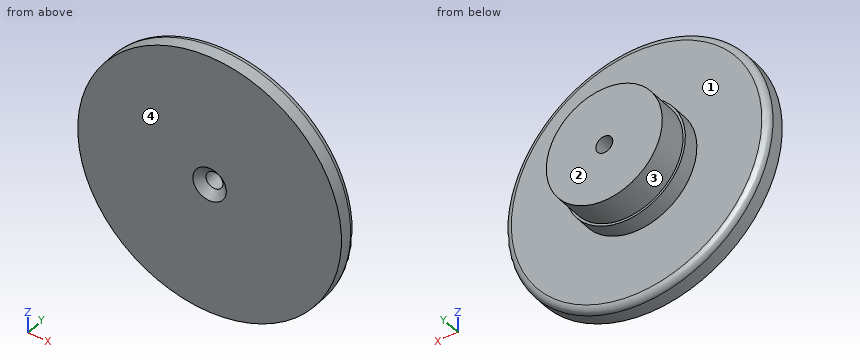
```python
from build123d import *

# Parameters (mm, degrees)
SKETCH1_R                                           = 50.8
SKETCH1_R_2                                         = 23.241
BOSS_EXTRUDE4_DEPTH                                 = 7.62
SKETCH1_6_R                                         = 23.241
SKETCH1_6_R_2                                       = 22.352
BOSS_EXTRUDE5_DEPTH                                 = 13.97
SKETCH1_7_R                                         = 22.352
BOSS_EXTRUDE6_DEPTH                                 = 25.4
CSK_FOR_1_4_FLAT_HEAD_MACHINE_SCREW_100_D           = 6.5278
CSK_FOR_1_4_FLAT_HEAD_MACHINE_SCREW_100_CSINK_D     = 12.8778
CSK_FOR_1_4_FLAT_HEAD_MACHINE_SCREW_100_CSINK_ANGLE = 100
FILLET3_R                                           = 2.54


with BuildPart() as part:
    # Sketch1 → Boss-Extrude4 (new body)
    with BuildSketch(Plane(origin=(0, 0, 0), x_dir=(1, 0, 0), z_dir=(0, 1, 0))):
        with Locations(Location((0, 0, 0), (0, 0, 90))):
            Circle(SKETCH1_R)
        with Locations(Location((0, 0, 0), (0, 0, 90))):
            Circle(SKETCH1_R_2, mode=Mode.SUBTRACT)
    extrude(amount=BOSS_EXTRUDE4_DEPTH)

    # Sketch1_6 → Boss-Extrude5 (add)
    with BuildSketch(Plane(origin=(0, 0, 0), x_dir=(1, 0, 0), z_dir=(0, 1, 0))):
        with Locations(Location((0, 0, 0), (0, 0, 270))):
            Circle(SKETCH1_6_R)
        with Locations(Location((0, 0, 0), (0, 0, 270))):
            Circle(SKETCH1_6_R_2, mode=Mode.SUBTRACT)
    extrude(amount=BOSS_EXTRUDE5_DEPTH)

    # Sketch1_7 → Boss-Extrude6 (add)
    with BuildSketch(Plane(origin=(0, 0, 0), x_dir=(1, 0, 0), z_dir=(0, 1, 0))):
        with Locations(Location((0, 0, 0), (0, 0, 270))):
            Circle(SKETCH1_7_R)
    extrude(amount=BOSS_EXTRUDE6_DEPTH)

    # CSK for 1_4 Flat Head Machine Screw _100 (through all)
    with Locations(Plane(origin=(0, 0, 0), x_dir=(-1, 0, 0), z_dir=(0, -1, 0))):
        with Locations((0, 0)):
            CounterSinkHole(CSK_FOR_1_4_FLAT_HEAD_MACHINE_SCREW_100_D / 2, CSK_FOR_1_4_FLAT_HEAD_MACHINE_SCREW_100_CSINK_D / 2, counter_sink_angle=CSK_FOR_1_4_FLAT_HEAD_MACHINE_SCREW_100_CSINK_ANGLE)

    # Fillet3
    fillet3_edges = [part.edges().sort_by_distance(p)[0] for p in [
        (0, 7.62, 50.8),
    ]]
    fillet(fillet3_edges, radius=FILLET3_R)


solid = part.part
```
Can you work these out from the model? Positions are in its coordinate system, mm. Face numbers are marked on the shaded views. A direction names the side the tool comes from. Coordinates: 2 decimals unless noted, no trailing zeros. Write each loop counter-clockwise with the first axis right and the second up, starting at its lowest first coordinate (ties: lowest second). Pieces come first, ordered by that corner, then holes. Notation, with made-up numbers: M 6.25,8 L 56.25,8 A22 ccw 56.25,44 Z; hole C 49.5,41.25 d6. An arc over 180 degrees is marked long. Write item = value, one per line. Start each with the question number.
Q1. Thinking about a two-plate mould opening in X: for the marked faces 3 and 4, which applies, released by +X, released by -X, zero draft, split by the parting line, or undercut?
Q2. I'm going to push flat-ended pins straight in: pin 1 (12 mm diameter, centred on x = -40, y = 6, fed in from -Z); pin 2 (4 mm diameter, centred on x = 36, y = 10.5, fed in from -Z); pin 3 (6 mm diameter, centred on x = -28.5, y = 7, fed in from +Z); pin 4 (12 mm diameter, centred on y = 4, z = -15, fed in from -X). Where does each tip first touch, or does it pass through?
Q3. If we section it at B-B, the plane z = 0: Write out the boundary of the cut face in (x, y), then the cut area to 3 significant figures.
Q4. If we section it at A-A, the plane x = 0: Write out the boundary of the cut face in (y, z).
Q5. On a 3-axis mill with a long thin cutter (end or side, diameter ignored), from which of +Z, -Z, +X, -X, +Y, -Y can I reach the whole of each face in a straight line? I mean the marked faces 1 and 2. Say none if no direction works.
Q6. If we section it at C-C, the plane y = 17: Write out the boundary of the cut face in (x, z).
Q7. If I drill on L1, parallel to Y at x = 42.5, z = -2.5; L2, parallel to X at y = 5.5, z = 1; L3, parallel to Z at x = -13.5, y = 10.75, over which ranges is the centre line in solid material (lowest first)? Write a range as [from, to].
Check sheet entries:
q1.face_3 = split by the parting line
q1.face_4 = zero draft
q2.pin_1 = -37.69
q2.pin_2 = through
q2.pin_3 = 43.67
q2.pin_4 = -50
q3.outline = M -50.8,0 L -6.44,0 L -3.26,2.66 L -3.26,25.4 L -22.35,25.4 L -22.35,13.97 L -23.24,13.97 L -23.24,7.62 L -48.26,7.62 A2.54 ccw -50.8,5.08 Z; M 3.26,2.66 L 6.44,0 L 50.8,0 L 50.8,5.08 A2.54 ccw 48.26,7.62 L 23.24,7.62 L 23.24,13.97 L 22.35,13.97 L 22.35,25.4 L 3.26,25.4 Z
q3.area = 1,400 mm²
q4.outline = M 0,-50.8 L 5.08,-50.8 A2.54 ccw 7.62,-48.26 L 7.62,-23.24 L 13.97,-23.24 L 13.97,-22.35 L 25.4,-22.35 L 25.4,-3.26 L 2.66,-3.26 L 0,-6.44 Z; M 0,6.44 L 2.66,3.26 L 25.4,3.26 L 25.4,22.35 L 13.97,22.35 L 13.97,23.24 L 7.62,23.24 L 7.62,48.26 A2.54 ccw 5.08,50.8 L 0,50.8 Z
q5.face_1 = +Y
q5.face_2 = +Z, -Z, +X, -X, +Y
q6.outline = C 0,0 d44.7; hole C 0,0 d6.53
q7.L1 = [0, 7.62]
q7.L2 = [-50.76, -3.11], [3.11, 50.76]
q7.L3 = [-18.92, 18.92]
